Work out the finished part from the listing and answer in its coordinate system (mm). Face numbers are marked on the shaded views. A direction names the side the tool comes from. Coordinates: 2 decimals unless noted, no trailing zeros. Order: outer loops, then holes, each group sorted by start corner. A loop starts at its lowest first (then second) coordinate and runs counter-clockwise, first axis right, second up. Notation, with made-up numbers: (7.25, 54.5) -> (54.25, 54.5) arc R25 ccw to (54.25, 91.5) -> close; hole circle Ø10 at (82, 11.5). An arc over 180 degrees is marked (long way). Use one line per item in the form item = value.
from build123d import *

# Parameters (mm, degrees)
BOSS_EXTRUDE1_DEPTH  = 1.5
SKETCH1_8_R          = 4.1
BOSS_EXTRUDE3_DEPTH  = 36
SKETCH1_9_R          = 5.05
BOSS_EXTRUDE4_DEPTH  = 19
SHELL1_START         = 2
SHELL1_OUTLINE_R     = 2.1
SHELL1_DEPTH         = 32
SHELL1_2_OUTLINE_R   = 3.05
SHELL1_2_OUTLINE_R_2 = 2.1
SHELL1_2_DEPTH       = 15
SKETCH1_10_R         = 3.25
CUT_EXTRUDE1_DEPTH   = 17
SKETCH1_3_R          = 3.25
BOSS_EXTRUDE2_DEPTH  = 6
CHAMFER1_SIZE        = 2
CHAMFER1_SIZE2       = 0.727940469
CHAMFER2_SIZE        = 2.747477419
CHAMFER2_SIZE_2      = 1
CHAMFER3_SIZE        = 1.212435565
CHAMFER3_SIZE_2      = 0.7
CHAMFER6_SIZE        = 0.3
FILLET1_R            = 3.2
CHAMFER5_SIZE        = 0.3
FILLET2_R            = 1
FILLET3_R            = 2


# Read off the part's stored shape, not the designer's step: Shell1
with BuildPart() as part:
    # Sketch1 → Boss-Extrude1 (new body)
    with BuildSketch(Plane.XY):
        Polygon((-10.6, 6.119912853), (0, 12.239825707), (10.6, 6.119912853), (10.6, -6.119912853), (0, -12.239825707), (-10.6, -6.119912853), align=None)
    extrude(amount=BOSS_EXTRUDE1_DEPTH)

    # Sketch1<8> → Boss-Extrude3 (add)
    with BuildSketch(Plane.XY):
        with Locations(Location((0, 0, 0), (0, 0, 180))):
            Circle(SKETCH1_8_R)
    extrude(amount=BOSS_EXTRUDE3_DEPTH)

    # Sketch1<9> → Boss-Extrude4 (add)
    with BuildSketch(Plane.XY):
        with Locations(Location((0, 0, 0), (0, 0, 180))):
            Circle(SKETCH1_9_R)
    extrude(amount=BOSS_EXTRUDE4_DEPTH)

    # Shell1 outline → Shell1 (cut)
    with BuildSketch(Plane.XY.offset(SHELL1_START)):
        Circle(SHELL1_OUTLINE_R)
    extrude(amount=SHELL1_DEPTH, mode=Mode.SUBTRACT)

    # Shell1 2 outline → Shell1 2 (cut)
    with BuildSketch(Plane.XY.offset(SHELL1_START)):
        Circle(SHELL1_2_OUTLINE_R)
        Circle(SHELL1_2_OUTLINE_R_2, mode=Mode.SUBTRACT)
    extrude(amount=SHELL1_2_DEPTH, mode=Mode.SUBTRACT)

    # Sketch1<10> → Cut-Extrude1 (cut)
    with BuildSketch(Plane.XY):
        Circle(SKETCH1_10_R)
    extrude(amount=CUT_EXTRUDE1_DEPTH, mode=Mode.SUBTRACT)

    # Sketch1<3> → Boss-Extrude2 (add)
    with BuildSketch(Plane.XY):
        Polygon((0, 11.200595222), (9.7, 5.600297611), (9.7, -5.600297611), (0, -11.200595222), (-9.7, -5.600297611), (-9.7, 5.600297611), align=None)
        Circle(SKETCH1_3_R, mode=Mode.SUBTRACT)
    extrude(amount=BOSS_EXTRUDE2_DEPTH)

    # Chamfer1
    chamfer1_edges = [part.edges().sort_by_distance(p)[0] for p in [
        (4.1, 0, 36),
    ]]
    chamfer1_side = [part.faces().sort_by_distance(p)[0] for p in [
        (4.1, 0, 27.5),
    ]]
    chamfer(chamfer1_edges, length=CHAMFER1_SIZE, length2=CHAMFER1_SIZE2, reference=chamfer1_side[0])

    # Chamfer2
    # the kernel refuses this chamfer: 2.747477419, 1 mm, written as the material it adds along each edge
    with BuildSketch(Plane(origin=(0, 0, 19), x_dir=(-1, 0, 0), z_dir=(0, -1, 0))) as chamfer2_piece_1_section:
        Polygon((4.1, -CHAMFER2_SIZE), (4.1 + CHAMFER2_SIZE_2, 0), (4.1, 0), align=None)
    chamfer2_piece_1 = revolve(axis=Axis((0, 0, 19), (0, 0, -1)), mode=Mode.PRIVATE)
    chamfer2_piece_1 = chamfer2_piece_1 & Plane(origin=(0, 0, 20.481947897), x_dir=(-1, 0, 0), z_dir=(0, 0, -1)) * Cylinder(5.05, 21, mode=Mode.PRIVATE)
    add(chamfer2_piece_1)

    # Chamfer3
    # the kernel refuses this chamfer: 1.212435565, 0.7 mm, written as the material it takes off along each edge
    with BuildSketch(Plane(origin=(0, 0, 17), x_dir=(1, 0, 0), z_dir=(0, -1, 0))) as chamfer3_piece_1_section:
        Polygon((2.1 + CHAMFER3_SIZE, 0), (2.1, CHAMFER3_SIZE_2), (2.1, 0), align=None)
    chamfer3_piece_1 = revolve(axis=Axis((0, 0, 17), (0, 0, 1)), mode=Mode.PRIVATE)
    chamfer3_piece_1 = chamfer3_piece_1 & Plane(origin=(0, 0, 17.363214185), x_dir=(1, 0, 0), z_dir=(0, 0, -1)) * Cylinder(3.25, 14, mode=Mode.PRIVATE)
    add(chamfer3_piece_1, mode=Mode.SUBTRACT)

    # Chamfer6
    chamfer6_edges = [part.edges().sort_by_distance(p)[0] for p in [
        (-3.25, 0, 0),
    ]]
    chamfer(chamfer6_edges, length=CHAMFER6_SIZE)

    # Fillet1
    fillet1_edges = [part.edges().sort_by_distance(p)[0] for p in [
        (-9.7, -5.600297611, 3.75),
        (0, -11.200595222, 3.75),
        (9.7, -5.600297611, 3.75),
        (9.7, 5.600297611, 3.75),
        (0, 11.200595222, 3.75),
        (-9.7, 5.600297611, 3.75),
    ]]
    fillet(fillet1_edges, radius=FILLET1_R)

    # Chamfer5
    chamfer5_edges = [part.edges().sort_by_distance(p)[0] for p in [
        (-4.85, -8.400446417, 6),
        (4.85, 8.400446417, 6),
        (-4.85, 8.400446417, 6),
        (-9.7, 0, 6),
        (9.271281292, 5.35277675, 6),
        (0, 10.705553499, 6),
        (-9.271281292, 5.35277675, 6),
        (-9.271281292, -5.35277675, 6),
        (0, -10.705553499, 6),
        (9.271281292, -5.35277675, 6),
        (5.3, 9.17986928, 1.5),
        (10.6, 0, 1.5),
        (5.3, -9.17986928, 1.5),
        (-5.3, -9.17986928, 1.5),
        (-10.6, 0, 1.5),
        (-5.3, 9.17986928, 1.5),
        (9.7, 0, 6),
        (4.85, -8.400446417, 6),
    ]]
    chamfer(chamfer5_edges, length=CHAMFER5_SIZE)

    # Fillet2
    fillet2_edges = [part.edges().sort_by_distance(p)[0] for p in [
        (10.6, 6.119912853, 0.6),
        (10.6, -6.119912853, 0.6),
        (0, -12.239825707, 0.6),
        (-10.6, -6.119912853, 0.6),
        (-10.6, 6.119912853, 0.6),
        (0, 12.239825707, 0.6),
    ]]
    fillet(fillet2_edges, radius=FILLET2_R)

    # Fillet3
    fillet3_edges = [part.edges().sort_by_distance(p)[0] for p in [
        (5.05, 0, 6),
    ]]
    fillet(fillet3_edges, radius=FILLET3_R)


solid = part.part
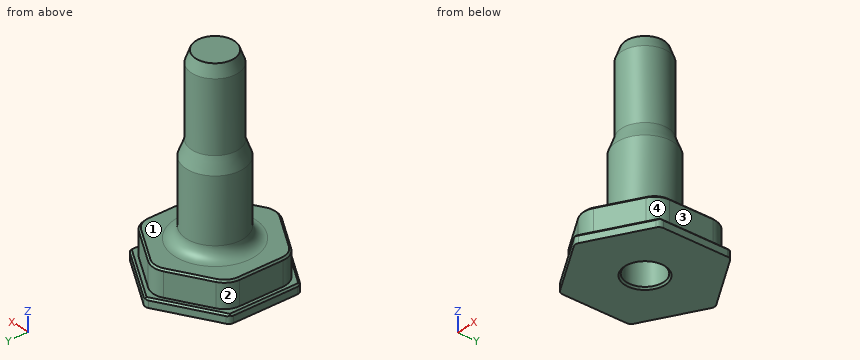
(1) Section C-C on z = 16 is taken. Write down the section's boundary in (x, y), plus the area to 3 significant figures.
Data:
outline = circle Ø10.1 at (0, 0); hole circle Ø6.5 at (0, 0)
area = 46.9 mm²
(2) Each of these flat-tipped pins is pushed along its axis until it touches: P1, Ø3.5, axis at x = 0, y = -1, coming from the -Z side; P2, Ø1.5, axis at x = 2, z = 14.5, coming from the +Y side; P3, Ø3.5, axis at y = 1.5, z = 4.5, coming from the -X side. Where does it stop, or does it pass through?
Data:
P1 = 17.32
P2 = 4.89
P3 = -9.7
(3) Section B-B on z = 3 is taken. Write down the section's boundary in (x, y), plus the area to 3 significant figures.
Data:
outline = (-9.7, -3.75) arc R3.2 ccw to (-8.1, -6.52) -> (-1.6, -10.28) arc R3.2 ccw to (1.6, -10.28) -> (8.1, -6.52) arc R3.2 ccw to (9.7, -3.75) -> (9.7, 3.75) arc R3.2 ccw to (8.1, 6.52) -> (1.6, 10.28) arc R3.2 ccw to (-1.6, 10.28) -> (-8.1, 6.52) arc R3.2 ccw to (-9.7, 3.75) -> close; hole circle Ø6.5 at (0, 0)
area = 289 mm²
(4) Which of the six approach directions +Z, -Z, +X, -X, +Y, -Y give full straight-line access (tool end or side, diameter ignored) to the marked faces 1, 2, 3 and 4?
Data:
face_1 = +Z
face_2 = +Z, -X, +Y
face_3 = +Z, +X, +Y, -Y
face_4 = +Z, +X, -Y
(5) Straight lines are drawn through the part: line 1 along Y through (x, z) = (0, 25.75); line 2 along Y through (x, z) = (0, 5); line 3 along Z through (x, y) = (0.75, -10). For each, find the intervals that lie inside material, in ascending order.
Data:
line_1 = -4.1 to -2.1, 2.1 to 4.1
line_2 = -10.71 to -3.25, 3.25 to 10.71
line_3 = 0 to 6
(6) Section D-D on y = -9.5 is taken. Write down the section's boundary in (x, z).
Data:
outline = (-4.75, 0) -> (4.75, 0) -> (4.75, 1.2) -> (4.15, 1.5) -> (2.95, 1.5) -> (2.95, 5.7) -> (2.35, 6) -> (-2.35, 6) -> (-2.95, 5.7) -> (-2.95, 1.5) -> (-4.15, 1.5) -> (-4.75, 1.2) -> close
